Build history of the part. All positions in model axes, mm. Give positions to 0.01 mm unless a question says otherwise; leave off trailing zeros. Loops run counter-clockwise (first coordinate to the right, second up) from the corner with the lowest first, then second, coordinate; pieces in that order, holes last. Notation, with made-up numbers: M 58.5,37.5 L 112.5,37.5 A11 ccw 112.5,58.5 Z; hole C 37.25,69 d3. An arc over 180 degrees is marked long. Put each result on its own line as item: value.
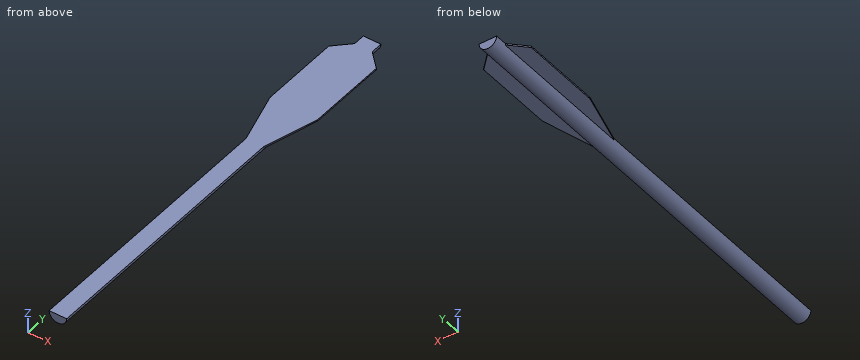
```python
from build123d import *

# Parameters (mm, degrees)
F1_DEPTH      = 144.5
F2_W          = 50
F2_H          = 0.5
F3_DEPTH      = 8
F3_DEPTH_BACK = 8
F4_DEPTH      = 0.5
F5_DEPTH      = 6
F6_DEPTH      = 0.5
F8_DEPTH      = 0.5


with BuildPart() as f1:
    # F0 (on Front) → F1 (new body)
    with BuildSketch(Plane.XZ):
        with BuildLine():
            ThreePointArc((-2.95, 0), (0, -2.95), (2.95, 0))
            Line((2.95, 0), (-2.95, 0))
        make_face()
    extrude(amount=F1_DEPTH)

    # F2 (on Right) → F3 (join, two sides)
    with BuildSketch(Plane.YZ) as f3_sk:
        with Locations((-29, 0.25)):
            Rectangle(F2_W, F2_H)
    extrude(amount=F3_DEPTH)
    extrude(f3_sk.sketch, amount=-F3_DEPTH_BACK)

    # F4 (add): faces of the model
    f4_faces = [f1.faces().sort_by_distance(p)[0] for p in [
        (5.475, -29, 0),
        (-5.475, -29, 0),
    ]]
    extrude(f4_faces, amount=F4_DEPTH)

    # F5 (add): a face of the model
    f5_faces = [f1.faces().sort_by_distance(p)[0] for p in [
        (-2.95, -29, -0.25),
    ]]
    extrude(f5_faces, amount=F5_DEPTH)

    # F6 (cut): a face of the model
    f6_faces = [f1.faces().sort_by_distance(p)[0] for p in [
        (0, -29, 0.5),
    ]]
    extrude(f6_faces, amount=-F6_DEPTH, mode=Mode.SUBTRACT)

    # F7 (on face) → F8 (cut)
    with BuildSketch(Plane.XY):
        Polygon((-8, -9), (-2.95, -4), (-8, -4), align=None)
        Polygon((-2.95, -54), (-8, -36), (-8, -54), align=None)
        Polygon((8, -54), (8, -36), (2.95, -54), align=None)
        Polygon((8, -4), (2.95, -4), (8, -9), align=None)
    extrude(amount=-F8_DEPTH, mode=Mode.SUBTRACT)


solid = f1.part
```
Q1. Slice it at A-A (y = -108.5). List the corners of the cut face in (x, z).
Here are the results:
outline: M -2.95,0 A2.95 ccw 2.95,0 Z
Q2. Drop flat-ended pins along their axis: pin 1 Ø5.5 at (x, y) = (-5, -23) entering from -Z; pin 2 Ø1.5 at (x, z) = (3, -1) entering from +Y; pin 3 Ø5.5 at (x, y) = (6, -41) entering from -Z; pin 4 Ø6 at (x, y) = (5.5, -23) entering from -Z. Give the stop position or say it passes through.
Here are the results:
pin 1: z = -1.91
pin 2: y = 0
pin 3: z = -0.5
pin 4: z = -1.57
Q3. Probe line 1 (X direction, y = -125.5, z = -0.3); line 2 (Z direction, x = -5, y = -7); line 3 (Z direction, x = -0.5, y = -63). List the from-to ranges inside material, lowest first. Write a range as from..to.
Here are the results:
line 1: -2.93..2.93
line 2: -0.5..0
line 3: -2.91..0
Q4. Slice it at C-C (z = -1.4). List the corners of the cut face in (x, y).
Here are the results:
outline: M -2.6,-144.5 L 2.6,-144.5 L 2.6,0 L -2.6,0 Z
Q5. Slice it at D-D (y = -15). List the corners of the cut face in (x, z).
Here are the results:
outline: M -8,-0.5 L -2.91,-0.5 A2.95 ccw 2.91,-0.5 L 8,-0.5 L 8,0 L -8,0 Z
Q6. Slice it at B-B (x = -5.5). List the corners of the cut face in (y, z).
Here are the results:
outline: M -44.91,-0.5 L -6.52,-0.5 L -6.52,0 L -44.91,0 Z
